The figure shows three views and two pictorial views of one solid part (mm, origin at its lowest corner). Answer the questions. Coordinates: 2 decimals unless noted, no trailing zeros. Order: outer loops, then holes, each group sorted by start corner. A loop starts at its lowest first (then second) coordinate and runs counter-clockwise, first axis right, second up. Notation, with made-up numbers: (6, 17) -> (21, 17) arc R9 ccw to (21, 23) -> close; hole circle Ø11 at (38, 10). An arc over 180 degrees is marked (long way). Write item = value, one per line.
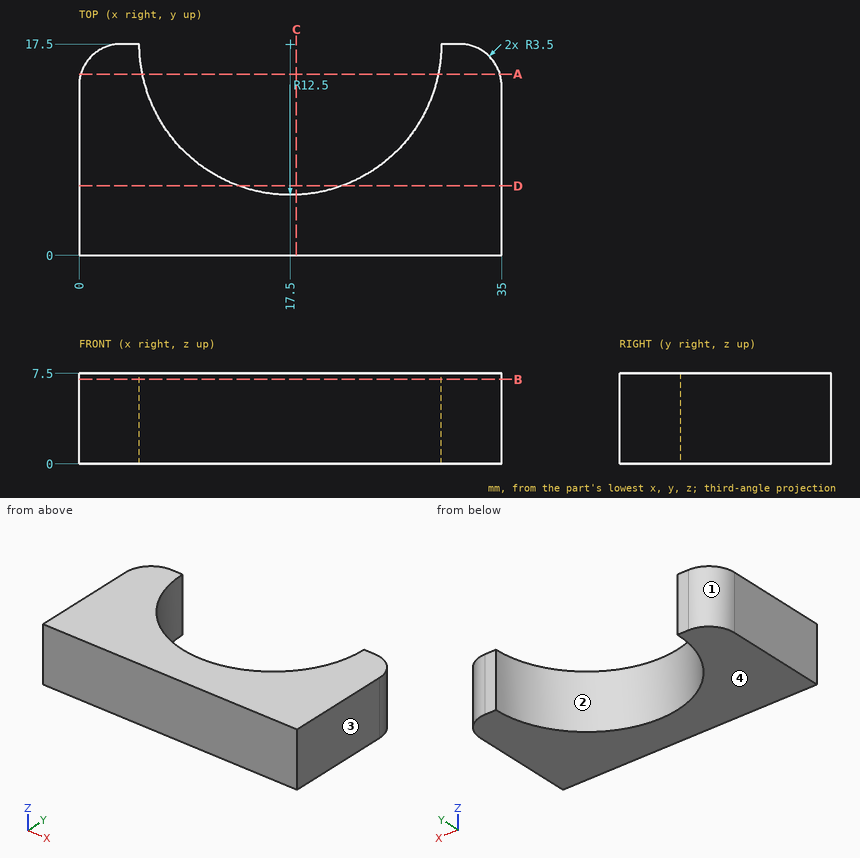
Q1. The mould has two halves that part along X. Classify the marked faces 1, 2, 3 and 4: released by +X, released by -X, zero draft, split by the parting line, or undercut.
The answers:
face_1 = released by -X
face_2 = undercut
face_3 = released by +X
face_4 = zero draft
Q2. Section B-B, the plane z = 7 is taken. Give the vertices of the cut face in (x, y), plus the area to 3 significant figures.
The answers:
outline = (0, 0) -> (35, 0) -> (35, 14) arc R3.5 ccw to (31.5, 17.5) -> (30, 17.5) arc R12.5 cw to (5, 17.5) -> (3.5, 17.5) arc R3.5 ccw to (0, 14) -> close
area = 362 mm2
Q3. Find the intervals of material crossed by line 1 along X through (y, z) = (7, 2); line 2 along X through (y, z) = (9.75, 4.5); line 3 along Y through (x, z) = (25, 1.5), in increasing order.
The answers:
line_1 = 0 to 10.72, 24.28 to 35
line_2 = 0 to 7.69, 27.31 to 35
line_3 = 0 to 7.5
Q4. Section A-A, the plane y = 15 is taken. Give the vertices of the cut face in (x, z), plus the area to 3 significant figures.
The answers:
outline = (0.15, 0) -> (5.25, 0) -> (5.25, 7.5) -> (0.15, 7.5) -> close; (29.75, 0) -> (34.85, 0) -> (34.85, 7.5) -> (29.75, 7.5) -> close
area = 76.6 mm2
Q5. Section C-C, the plane x = 18 is taken. Give the vertices of the cut face in (y, z).
The answers:
outline = (0, 0) -> (5.01, 0) -> (5.01, 7.5) -> (0, 7.5) -> close
Q6. Each of these flat-tipped pins is pushed along its axis until it touches: pin 1 Ø2 at (x, z) = (17, 5.5) entering from +Y; pin 2 Ø1 at (x, z) = (6.5, 5) entering from +Y. Where does it stop, or does it pass through?
The answers:
pin_1 = 5.09
pin_2 = 12.6
Q7. Section D-D, the plane y = 5.75 is taken. Give the vertices of the cut face in (x, z).
The answers:
outline = (0, 0) -> (13.24, 0) -> (13.24, 7.5) -> (0, 7.5) -> close; (21.76, 0) -> (35, 0) -> (35, 7.5) -> (21.76, 7.5) -> close
